```python
from build123d import *

# Parameters (mm, degrees)
BOSS_EXTRUDE1_DEPTH = 302.625
SKETCH3_W           = 760
SKETCH3_H           = 10
BOSS_EXTRUDE2_DEPTH = 50
SKETCH4_W           = 760
SKETCH4_H           = 10
BOSS_EXTRUDE3_DEPTH = 50


with BuildPart() as part:
    # Sketch2 → Boss-Extrude1 (new body, symmetric)
    with BuildSketch(Plane.XY):
        Polygon((0, 25), (-380, 25), (-380, 15), (-225, 15), (-225, 0), (0, 0), align=None)
    boss_extrude1 = extrude(amount=BOSS_EXTRUDE1_DEPTH, both=True)

    # Mirror1: Boss-Extrude1 across plane
    add(boss_extrude1.mirror(Plane(origin=(0, 25, 302.625), x_dir=(0, 0, 1), z_dir=(-1, 0, 0))))

    # Sketch3 → Boss-Extrude2 (add)
    with BuildSketch(Plane.XY.offset(302.625)):
        with Locations((0, 20)):
            Rectangle(SKETCH3_W, SKETCH3_H)
    extrude(amount=BOSS_EXTRUDE2_DEPTH)

    # Sketch4 → Boss-Extrude3 (add)
    with BuildSketch(Plane(origin=(0, 0, -302.625), x_dir=(-1, 0, 0), z_dir=(0, 0, -1))):
        with Locations((0, 20)):
            Rectangle(SKETCH4_W, SKETCH4_H)
    extrude(amount=BOSS_EXTRUDE3_DEPTH)


solid = part.part
```
The listing builds one solid part. Answer for the finished solid, in the listing's coordinates (mm). Coordinates: 2 decimals unless noted, no trailing zeros. Write each loop counter-clockwise with the first axis right and the second up, starting at its lowest first coordinate (ties: lowest second). Pieces come first, ordered by that corner, then holes. Notation, with made-up numbers: (12.25, 54) -> (17.25, 54) arc R11 ccw to (17.25, 62) -> close; hole circle Ø6 at (52, 11). An arc over 180 degrees is marked (long way). Write each question's results on one line, items separated by ' | '. Start each with the question number.
1) A cutting plane is placed at B-B (z = -225.5). Determine the outline of the cut face in (x, y).
2) Flat-ended cylindrical pins translate along their axes: pin 1 Ø4.5 at (y, z) = (4.5, 0.5) entering from -X; pin 2 Ø4.5 at (y, z) = (6, -116.5) entering from +X; pin 3 Ø7.5 at (x, y) = (11.5, 4) entering from -Z (3 decimals). Find the tip coordinate at first contact, or state that the pin passes through.
3) Straight lines are drawn through the part: probe 1 along Z at (x, y) = (-35.5, 10) (3 decimals); probe 2 along X at (y, z) = (10.75, 81); probe 3 along Y at (x, z) = (-332.5, -83.5). For each, find the intervals that lie inside material, in ascending order.
4) A cutting plane is placed at D-D (x = -239.5). Determine the outline of the cut face in (y, z) (3 decimals).
5) A cutting plane is placed at A-A (x = -122). Determine the outline of the cut face in (y, z) (3 decimals).
6) A cutting plane is placed at C-C (y = 11). Determine the outline of the cut face in (x, z) (3 decimals).
Values follow:
1) outline: (-380, 15) -> (-225, 15) -> (-225, 0) -> (225, 0) -> (225, 15) -> (380, 15) -> (380, 25) -> (-380, 25) -> close
2) pin 1: x = -225 | pin 2: x = 225 | pin 3: z = -302.625
3) probe 1: -302.625 to 302.625 | probe 2: -225 to 225 | probe 3: 15 to 25
4) outline: (15, -352.625) -> (25, -352.625) -> (25, 352.625) -> (15, 352.625) -> close
5) outline: (0, -302.625) -> (15, -302.625) -> (15, -352.625) -> (25, -352.625) -> (25, 352.625) -> (15, 352.625) -> (15, 302.625) -> (0, 302.625) -> close
6) outline: (-225, -302.625) -> (225, -302.625) -> (225, 302.625) -> (-225, 302.625) -> close
